```python
from build123d import *

# Parameters (mm, degrees)
SKETCH1_R           = 4.99999
SKETCH1_R_2         = 2.182749
SKETCH1_R_3         = 2.0828
SKETCH1_R_4         = 1.932813
SKETCH1_R_5         = 1.732788
BOSS_EXTRUDE2_DEPTH = 4.99999
SKETCH1_5_R         = 2.0828
BOSS_EXTRUDE3_DEPTH = 107.999884076
BOSS_EXTRUDE4_START = -107.999884
SKETCH1_6_R         = 1.932813
BOSS_EXTRUDE4_DEPTH = 0.199898
BOSS_EXTRUDE5_START = -108.199782
SKETCH1_7_R         = 1.732788
BOSS_EXTRUDE5_DEPTH = 1.199896
BOSS_EXTRUDE6_START = -109.399678
SKETCH1_8_R         = 2.0828
BOSS_EXTRUDE6_DEPTH = 14.99997
CHAMFER1_SIZE       = 0.2032
CHAMFER2_SIZE       = 0.1905


with BuildPart() as part:
    # Sketch1 → Boss-Extrude2 (new body)
    # profile 1 of 5: a face of its own
    with BuildSketch(Plane(origin=(0, 0, 0), x_dir=(0, 0, -1), z_dir=(1, 0, 0))):
        Circle(SKETCH1_R)
        Circle(SKETCH1_R_2, mode=Mode.SUBTRACT)
    # profile 2 of 5: a face of its own
    with BuildSketch(Plane(origin=(0, 0, 0), x_dir=(0, 0, -1), z_dir=(1, 0, 0))):
        Circle(SKETCH1_R_2)
        Circle(SKETCH1_R_3, mode=Mode.SUBTRACT)
    # profile 3 of 5: a face of its own
    with BuildSketch(Plane(origin=(0, 0, 0), x_dir=(0, 0, -1), z_dir=(1, 0, 0))):
        Circle(SKETCH1_R_3)
        Circle(SKETCH1_R_4, mode=Mode.SUBTRACT)
    # profile 4 of 5: a face of its own
    with BuildSketch(Plane(origin=(0, 0, 0), x_dir=(0, 0, -1), z_dir=(1, 0, 0))):
        Circle(SKETCH1_R_4)
        Circle(SKETCH1_R_5, mode=Mode.SUBTRACT)
    # profile 5 of 5: a face of its own
    with BuildSketch(Plane(origin=(0, 0, 0), x_dir=(0, 0, -1), z_dir=(1, 0, 0))):
        Circle(SKETCH1_R_5)
    extrude(amount=-BOSS_EXTRUDE2_DEPTH)

    # Sketch1<5> → Boss-Extrude3 (add)
    with BuildSketch(Plane(origin=(0, 0, 0), x_dir=(0, 0, -1), z_dir=(1, 0, 0))):
        Circle(SKETCH1_5_R)
    extrude(amount=-BOSS_EXTRUDE3_DEPTH)

    # Sketch1<6> → Boss-Extrude4 (add)
    with BuildSketch(Plane(origin=(0, 0, 0), x_dir=(0, 0, -1), z_dir=(1, 0, 0)).offset(BOSS_EXTRUDE4_START)):
        Circle(SKETCH1_6_R)
    extrude(amount=-BOSS_EXTRUDE4_DEPTH)

    # Sketch1<7> → Boss-Extrude5 (add)
    with BuildSketch(Plane(origin=(0, 0, 0), x_dir=(0, 0, -1), z_dir=(1, 0, 0)).offset(BOSS_EXTRUDE5_START)):
        Circle(SKETCH1_7_R)
    extrude(amount=-BOSS_EXTRUDE5_DEPTH)

    # Sketch1<8> → Boss-Extrude6 (add)
    with BuildSketch(Plane(origin=(0, 0, 0), x_dir=(0, 0, -1), z_dir=(1, 0, 0)).offset(BOSS_EXTRUDE6_START)):
        Circle(SKETCH1_8_R)
    extrude(amount=-BOSS_EXTRUDE6_DEPTH)

    # Chamfer1
    # the kernel refuses this chamfer: 0.2032 mm, written as the material it takes off along each edge
    with BuildSketch(Plane(origin=(-108.199782, 0, 0), x_dir=(0, 0, -1), z_dir=(0, -1, 0))) as chamfer1_piece_1_section:
        Polygon((1.932813 - CHAMFER1_SIZE, 0), (1.932813, CHAMFER1_SIZE), (1.932813, 0), align=None)
    chamfer1_piece_1 = revolve(axis=Axis((-108.199782, 0, 0), (1, 0, 0)), mode=Mode.PRIVATE)
    chamfer1_piece_1 = chamfer1_piece_1 - Plane(origin=(-108.102785336, 0, 0), x_dir=(0, 0, -1), z_dir=(1, 0, 0)) * Cylinder(1.732788, 8, mode=Mode.PRIVATE)
    chamfer1_piece_1 = split(chamfer1_piece_1, bisect_by=Plane(origin=(-107.999884076, 0, 1.83568926), z_dir=(-1, 0, 0)), keep=Keep.TOP, mode=Mode.PRIVATE)
    add(chamfer1_piece_1, mode=Mode.SUBTRACT)

    # Chamfer2
    chamfer2_edges = [part.edges().sort_by_distance(p)[0] for p in [
        (-124.399648, 0, 2.0828),
    ]]
    chamfer(chamfer2_edges, length=CHAMFER2_SIZE)


solid = part.part
```
CAD build for the part. Positions are in the model's coordinates, mm. A direction names the side the tool comes from. Coordinates: 2 decimals unless noted, no trailing zeros. Order: outer loops, then holes, each group sorted by start corner. A loop starts at its lowest first (then second) coordinate and runs counter-clockwise, first axis right, second up. Notation, with made-up numbers: (-27.75, -38.75) - (6.25, -38.75) arc R21 ccw to (6.25, -6.75) - close; hole circle Ø7 at (40.25, -24). An arc over 180 degrees is marked (long way). Use a Markdown table: item, result. Add a question column.
(1) Saw through at A-A (z = 0). Give the cut face in (x, y), then the cut area to 3 significant figures.
(2) Flat gauge pins, fed straight in: pin 1 (1.5 mm diameter, centred on x = -109.5, y = -0.5, fed in from +Z); pin 2 (3 mm diameter, centred on x = -83.5, y = -2.5, fed in from +Z); pin 3 (3 mm diameter, centred on y = 0, z = -2.5, fed in from +X); pin 4 (3 mm diameter, centred on x = -68.5, y = 2.5, fed in from -Z). Where does each tip first touch, or does it go through?
(3) Which spindle directions (+Z, -Z, +X, -X, +Y, -Y) get a long thin tool onto all of the face, cutting with end or side? Do faces 4 (the face through (-5, -2, -1)), 5 (the face through (-124.4, 0, 0)). Say none if no direction does.
(4) Pull direction X, two halves, no side cores. Call faces 1 (the face through (0, 0, 0)), 2 (the face through (-108.79, 0.08, 1.73)), 3 (the face through (-116.701, 0.626, -1.987)): +X half, -X half, draft (parallel to the pull), parting line (faces both ways), or undercut.
(5) Saw through at C-C (x = -80.5). Give the cut face in (y, z).
(6) Drill centre lines: line 1 along X through (y, z) = (-2, -3.25); line 2 along Y through (x, z) = (-73.5, 0.25). Where is each one in solid material? Low to high. Write a range as [from, to].
Solved:
| question | item | result |
|---|---|---|
| 1 | outline | (-124.4, -1.89) - (-124.21, -2.08) - (-109.4, -2.08) - (-109.4, -1.73) - (-108.2, -1.73) - (-108, -1.93) - (-108, -2.08) - (-5, -2.08) - (-5, -5) - (0, -5) - (0, 5) - (-5, 5) - (-5, 2.08) - (-108, 2.08) - (-108, 1.93) - (-108.2, 1.73) - (-109.4, 1.73) - (-109.4, 2.08) - (-124.21, 2.08) - (-124.4, 1.89) - close |
| 1 | area | 546 mm² |
| 2 | pin 1 | stops at z = 2.08 |
| 2 | pin 2 | stops at z = 1.83 |
| 2 | pin 3 | stops at x = 0 |
| 2 | pin 4 | stops at z = -1.83 |
| 3 | face 4 | -X |
| 3 | face 5 | +Z, -Z, -X, +Y, -Y |
| 4 | face 1 | +X half |
| 4 | face 2 | undercut |
| 4 | face 3 | draft |
| 5 | outline | circle Ø4.17 at (0, 0) |
| 6 | line 1 | x = [-5, 0] |
| 6 | line 2 | y = [-2.07, 2.07] |
